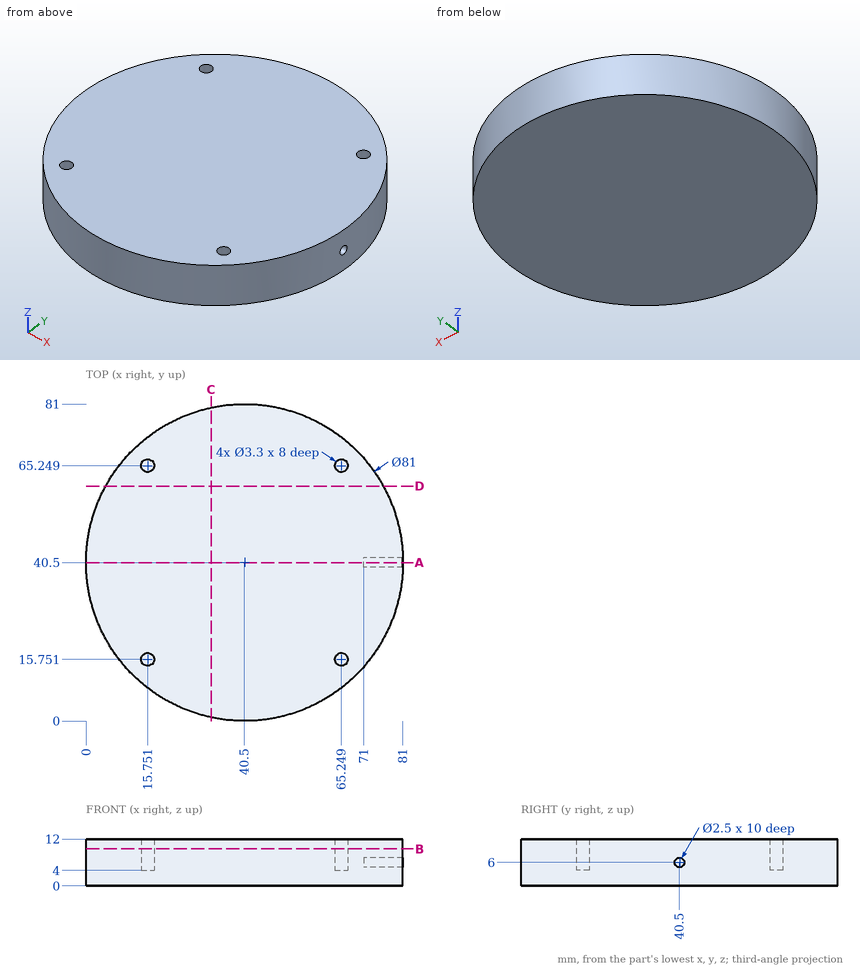
Input: dimensioned drawing with shaded views. Units: mm. Origin: part minimum x, y, z. Give positions to 0.01 mm unless a question says otherwise; leave off trailing zeros. Write each loop counter-clockwise with the first axis right and the second up, starting at its lowest first coordinate (ties: lowest second). Pieces come first, ordered by that corner, then holes.
1. Section query D-D, the plane y = 60. Return loops of the section in (x, z).
2. Section query A-A, the plane y = 40.5. Return loops of the section in (x, z).
3. Pin query (flat end, axial travel): P1, Ø1.6, axis at x = 15.5, y = 15.5, coming from the +Z side; P2, Ø3, axis at x = 40.5, z = 4.5, coming from the -Y side; P3, Ø3, axis at y = 24, z = 6.5, coming from the +X side. Return the tip coordinate at first contact, or that it passes through.
4. Section query C-C, the plane x = 32. Return loops of the section in (y, z).
5. Section query B-B, the plane z = 9.5. Return loops of the section in (x, y), then the cut area to 3 significant figures.
6. Line query: probe 1 along Z at (x, y) = (78, 40.5); probe 2 along X at (y, z) = (66, 11.75) (1 decimal); probe 3 along Y at (x, z) = (16.5, 4.5). Output: solid intervals per line, ascending.
Computed:
1. outline: (5, 0) - (76, 0) - (76, 12) - (5, 12) - close
2. outline: (0, 0) - (81, 0) - (81, 4.75) - (71, 4.75) - (71, 7.25) - (81, 7.25) - (81, 12) - (0, 12) - close
3. P1: stops at z = 4
3. P2: stops at y = 0
3. P3: stops at x = 78.12
4. outline: (0.9, 0) - (80.1, 0) - (80.1, 12) - (0.9, 12) - close
5. outline: circle Ø81 at (40.5, 40.5); hole circle Ø3.3 at (15.75, 15.75); hole circle Ø3.3 at (15.75, 65.25); hole circle Ø3.3 at (65.25, 15.75); hole circle Ø3.3 at (65.25, 65.25)
5. area: 5,120 mm2
6. probe 1: z = 0 to 4.75, 7.25 to 12
6. probe 2: x = 9 to 14.3, 17.2 to 63.8, 66.7 to 72
6. probe 3: y = 7.88 to 14.28, 17.22 to 63.78, 66.72 to 73.12
